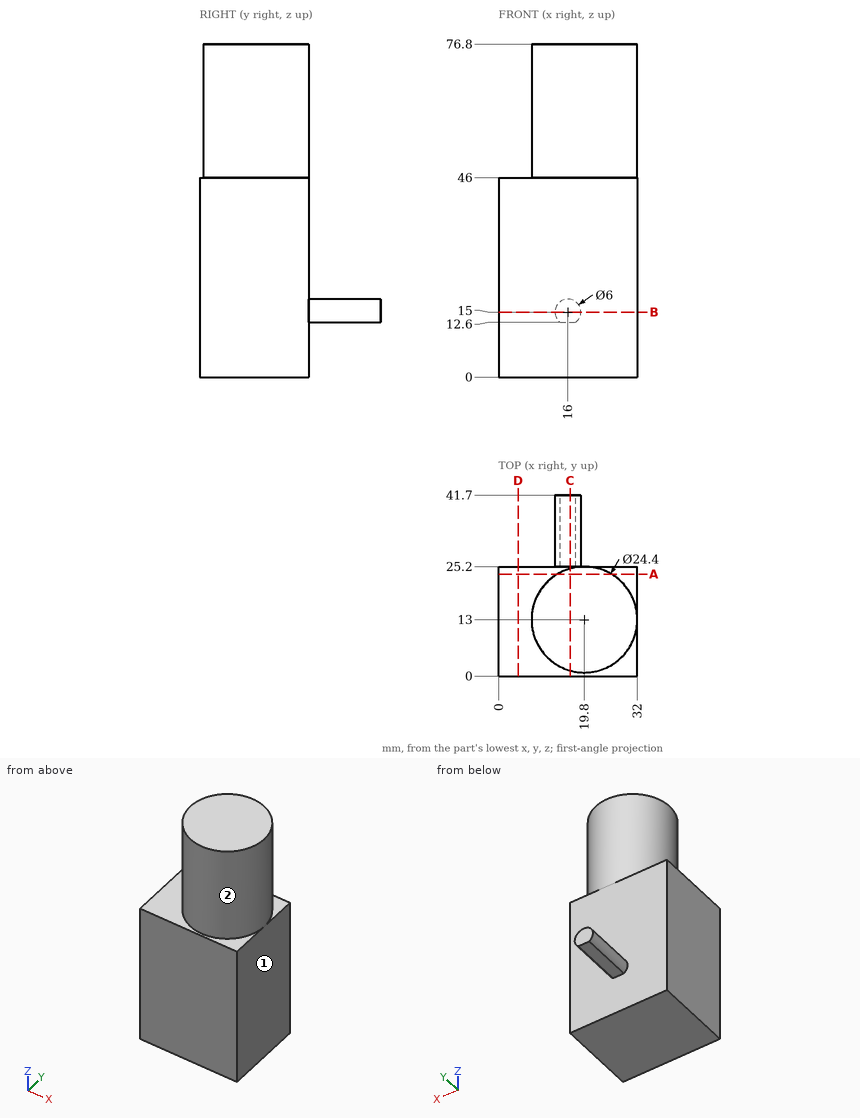
Can you work these out from the drawing? Everything is in mm from the part's minimum corner. A direction names the side the tool comes from. Coordinates: 2 decimals unless noted, no trailing zeros. Loops run counter-clockwise (first coordinate to the right, second up) from the corner with the lowest first, then second, coordinate; pieces in that order, holes last. Notation, with made-up numbers: M 14,58 L 41,58 A15 cw 41,64 Z; hole C 12.25,-34 d8. An arc over 180 degrees is marked long. Put each result on its own line as item: value. Start each with the question number.
(1) For the marked faces 1 and 2, which set-ups out of +Z, -Z, +X, -X, +Y, -Y let a thin tool reach every point of the face, with its end or its side?
(2) Suppose I cut it at C-C on x = 16.5. Please give me the cut outline in (y, z).
(3) Suppose I cut it at D-D on x = 4.5. Please give me the cut outline in (y, z).
(4) Suppose I cut it at B-B on z = 15. Please give me the cut outline in (x, y).
(5) Will these pins go through, and if not, where does the flat tip stop? P1, Ø1.5, axis at x = 19, z = 19, coming from the +Y side; P2, Ø3, axis at x = 16, y = 34.5, coming from the -Z side; P3, Ø1, axis at y = 15, z = 66, coming from the -X side.
(6) Suppose I cut it at A-A on y = 23.5. Please give me the cut outline in (x, z).
(7) I need wall thicknesses on line 1 (Y direction, x = 21, z = 38); line 2 (Z direction, x = 14, y = 25); line 3 (Y direction, x = 18, z = 62.5). Which ranges of each line are inside material? Lowest first, please. Write a range as from..to.
Solutions:
1. face 1: +Z, -Z, +X, +Y, -Y
1. face 2: +Z
2. outline: M 0,0 L 25.2,0 L 25.2,12.6 L 41.7,12.6 L 41.7,17.96 L 25.2,17.96 L 25.2,46 L 24.75,46 L 24.75,76.8 L 1.25,76.8 L 1.25,46 L 0,46 Z
3. outline: M 0,0 L 25.2,0 L 25.2,46 L 0,46 Z
4. outline: M 0,0 L 32,0 L 32,25.2 L 19,25.2 L 19,41.7 L 13,41.7 L 13,25.2 L 0,25.2 Z
5. P1: stops at y = 25.2
5. P2: stops at z = 12.6
5. P3: stops at x = 7.69
6. outline: M 0,0 L 32,0 L 32,46 L 26.01,46 L 26.01,76.8 L 13.59,76.8 L 13.59,46 L 0,46 Z
7. line 1: y = 0..25.2
7. line 2: z = 0..46
7. line 3: y = 0.93..25.07
